Can you work these out from the model? Positions are in its coordinate system, mm. Give positions to 0.01 mm unless a question says otherwise; leave off trailing zeros. Order: outer loops, then holes, each group sorted by start corner. A loop starts at its lowest first (then second) coordinate and runs counter-clockwise, first axis right, second up. Notation, with made-up numbers: M 7,-31.75 L 56,-31.75 A17 ccw 56,-14.75 Z; hole C 82.25,5.5 d11. An arc over 180 degrees is marked long. Write each question's results on one line, items separated by ' | '.
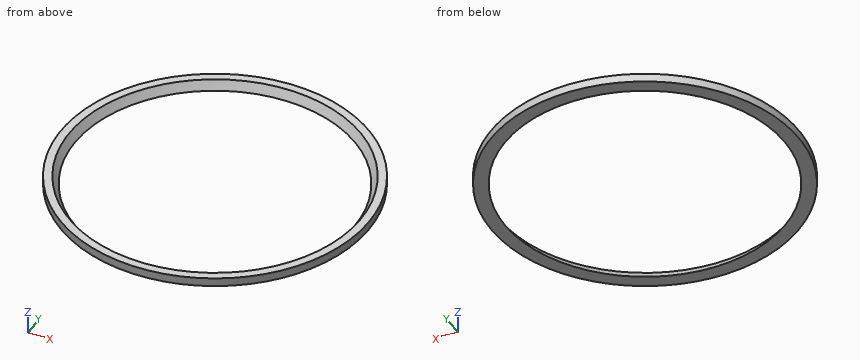
from build123d import *

# Parameters (mm, degrees)
SKETCH_R  = 18
PAD_DEPTH = 1


with BuildPart() as sphere:
    # Sphere → Sphere (revolve)
    with BuildSketch(Plane(origin=(0, 0, 11.5), x_dir=(1, 0, 0), z_dir=(0, -1, 0))):
        with BuildLine():
            ThreePointArc((0, -20), (20, 0), (0, 20))
            Line((0, 20), (0, -20))
        make_face()
    revolve(axis=Axis((0, 0, 11.5), (0, 0, 1)))


with BuildPart() as cut:
    # Sketch → Pad (new body)
    with BuildSketch(Plane.XY):
        Circle(SKETCH_R)
    extrude(amount=PAD_DEPTH)

    # Cut: cut Sphere
    add(sphere.part, mode=Mode.SUBTRACT)


solid = cut.part
(1) I need wall thicknesses on L1, parallel to Y at x = -1, z = 0.2; L2, parallel to X at y = -3, z = 0.65; L3, parallel to X at y = 11.5, z = 0.55. Which ranges of each line are inside material? Lowest first, please. Write a range as from..to.
Data:
L1: y = -17.97..-16.47, 16.47..17.97 | L2: x = -17.75..-16.53, 16.53..17.75 | L3: x = -13.85..-12.16, 12.16..13.85
(2) Imagine slicing it at B-B, the plane x = 0. Write out the boundary of the cut face in (y, z).
Data:
outline: M -18,0 L -16.36,0 A20 cw -17.02,1 L -18,1 Z; M 16.36,0 L 18,0 L 18,1 L 17.02,1 A20 cw Z
(3) Imagine slicing it at C-C, the plane z = 0.75. Write out the boundary of the cut face in (x, y), plus the area to 3 significant figures.
Data:
outline: C 0,0 d36; hole C 0,0 d33.73 | area: 124 mm2
(4) Imagine slicing it at A-A, the plane y = 11.5. Write out the boundary of the cut face in (x, z).
Data:
outline: M -13.85,0 L -11.64,0 A16.36 cw -12.55,1 L -13.85,1 Z; M 11.64,0 L 13.85,0 L 13.85,1 L 12.55,1 A16.36 cw Z
(5) Will these pins go through, and if not, where does the flat tip stop? P1, Ø2, axis at x = 13.5, y = 7.5, coming from the -Z side; P2, Ø5, axis at x = 13, y = 1.5, coming from the -Z side.
Data:
P1: stops at z = 0 | P2: passes through
